Work out the finished part from the listing and answer in its coordinate system (mm). A direction names the side the tool comes from. Coordinates: 2 decimals unless noted, no trailing zeros. Write each loop counter-clockwise with the first axis right and the second up, starting at its lowest first coordinate (ties: lowest second). Pieces come first, ordered by that corner, then holes. Notation, with made-up numbers: (53, 31) - (97, 31) arc R29 ccw to (97, 54) - close; hole circle Ø2 at (40.5, 77). An arc over 180 degrees is marked (long way). Use a Markdown table: item, result. Add a question column.
(1) For a pull along Y with two mould halves and no side action, classify faces 3 (the face through (-0.1, 22.2, 2.5)), 4 (the face through (0, 36.656, 0)), 5 (the face through (-1.15, 4.51, 0.15)) as released by +Y, released by -Y, zero draft, split by the parting line, or undercut.
(2) Find the intervals of material crossed by line 1 (Z direction, x = 0.15, y = 21); line 2 (X direction, y = 27.5, z = 0.2); line 3 (Z direction, x = 1, y = 30), in increasing order. Write a range as from..to.
(3) Given pin 1 Ø1 at (x, z) = (0, -1.5) entering from -Y, flat-ended and moving along its own axis, determine where the tip first touches the part or whether it passes through.
(4) The part is cut by section A-A, the plane y = 13.5. Give the vertices of the cut face in (x, z), then the cut area to 3 significant figures.
(5) A tool of negligible diameter and unlimited length cuts with its end or side. For faces 1 (the face through (-0.395, 2.233, -1.254)), 2 (the face through (0, 0, 0)), from which of +Z, -Z, +X, -X, +Y, -Y can it reach the whole face along a straight path? Write none if from no direction.
from build123d import *


with BuildPart() as part:
    # Sketch1 → Revolve3 (revolve)
    with BuildSketch(Plane.XY, mode=Mode.PRIVATE) as revolve3_sk:
        with BuildLine():
            Line((0, 0), (1.19724359, 0.09030412))
            ThreePointArc((1.19724359, 0.09030412), (1.403333579, 0.195244703), (1.473538086, 0.415601089))
            Line((1.473538086, 0.415601089), (1.159943816, 4))
            Line((1.159943816, 4), (1.159943816, 5))
            Line((1.159943816, 5), (2.5, 7.321045395))
            Line((2.5, 7.321045395), (2.5, 36.656450649))
            Line((2.5, 36.656450649), (0, 36.656450649))
            Line((0, 36.656450649), (0, 0))
        make_face()
    revolve(revolve3_sk.sketch.rotate(Axis((0, 0, 0), (0, 1, 0)), 90), axis=Axis((0, 0, 0), (0, 1, 0)))  # turned: the seam where the file's is


solid = part.part
Model answer:
| question | item | result |
|---|---|---|
| 1 | face 3 | zero draft |
| 1 | face 4 | released by +Y |
| 1 | face 5 | undercut |
| 2 | line 1 | -2.5..2.5 |
| 2 | line 2 | -2.49..2.49 |
| 2 | line 3 | -2.29..2.29 |
| 3 | pin 1 | y = 0.08 |
| 4 | outline | circle Ø5 at (0, 0) |
| 4 | area | 19.6 mm^2 |
| 5 | face 1 | none |
| 5 | face 2 | -Y |
